from build123d import *

# Parameters (mm, degrees)
F0_R     = 8
F1_DEPTH = 3.5
F2_R     = 12.5
F2_R_2   = 8
F3_DEPTH = 1
F4_W     = 20
F4_H     = 2
F5_DEPTH = 2
F6_W     = 1.5
F6_H     = 3
F7_DEPTH = 0.25


with BuildPart() as f1:
    # F0 (on Top) → F1 (new body)
    with BuildSketch(Plane.XY):
        with BuildLine():
            ThreePointArc((0, -12.5), (8.838835, -8.838835), (12.5, 0))
            ThreePointArc((12.5, 0), (8.838835, 8.838835), (0, 12.5))
            ThreePointArc((0, 12.5), (-12.5, 0), (0, -12.5))
        make_face()
        Circle(F0_R, mode=Mode.SUBTRACT)
        with BuildLine():
            ThreePointArc((0, -12.5), (-12.5, 0), (0, 12.5))
            Line((0, 12.5), (-35, 12.5))
            Line((-35, 12.5), (-116.388784, 2.506714))
            Line((-116.388784, 2.506714), (-116.388784, -2.506714))
            Line((-116.388784, -2.506714), (-35, -12.5))
            Line((-35, -12.5), (0, -12.5))
        make_face()
    extrude(amount=F1_DEPTH)

    # F2 (on face) → F3 (join)
    with BuildSketch(Plane.XY.offset(3.5)):
        Circle(F2_R)
        Circle(F2_R_2, mode=Mode.SUBTRACT)
    extrude(amount=F3_DEPTH)

    # F4 (on face) → F5 (cut)
    with BuildSketch(Plane.XY.offset(3.5)):
        with Locations((-106.388784, -0.006714)):
            Rectangle(F4_W, F4_H)
    extrude(amount=-F5_DEPTH, mode=Mode.SUBTRACT)

    # F6 (on face) → F7 (join)
    with BuildSketch(Plane.XY.offset(4.5)):
        with Locations((0, 10.153166)):
            Rectangle(F6_W, F6_H)
        Polygon((3.237552, 11.219494), (1.772621, 11.541949), (1.127709, 8.612088), (2.59264, 8.289632), align=None)
        Polygon((5.573719, 10.26121), (4.212356, 10.891044), (2.952689, 8.168318), (4.314052, 7.538484), align=None)
        Polygon((7.649265, 8.823124), (6.455126, 9.730885), (4.639603, 7.342606), (5.833743, 6.434845), align=None)
        Polygon((9.367141, 6.972478), (8.396061, 8.115721), (6.109575, 6.173563), (7.080655, 5.030319), align=None)
        Polygon((10.647019, 4.795807), (9.944406, 6.121075), (7.29387, 4.71585), (7.996483, 3.390582), align=None)
        Polygon((11.429054, 2.39489), (11.027762, 3.840215), (8.137112, 3.03763), (8.538404, 1.592305), align=None)
        Polygon((11.67668, -0.11801), (11.595471, 1.37979), (8.599871, 1.217373), (8.68108, -0.280427), align=None)
        Polygon((11.378317, -2.625392), (11.62099, -1.145153), (8.66051, -0.659807), (8.417837, -2.140046), align=None)
        Polygon((10.547916, -5.010014), (11.103124, -3.616549), (8.316193, -2.506134), (7.760986, -3.899599), align=None)
        Polygon((9.224307, -7.160373), (10.066088, -5.918839), (7.583021, -4.235278), (6.74124, -5.476812), align=None)
        Polygon((7.469379, -8.975921), (8.558373, -7.944371), (6.495274, -5.766385), (5.406281, -6.797934), align=None)
        Polygon((5.365192, -10.371764), (6.650478, -9.598434), (5.103816, -7.027862), (3.81853, -7.801193), align=None)
        Polygon((3.010134, -11.282636), (4.431614, -10.803684), (3.473709, -7.960724), (2.052229, -8.439676), align=None)
        Polygon((0.514325, -11.665944), (2.005532, -11.503765), (1.681175, -8.521352), (0.189968, -8.68353), align=None)
        Polygon((-2.005532, -11.503765), (-0.514325, -11.665944), (-0.189968, -8.68353), (-1.681175, -8.521352), align=None)
        Polygon((-4.431614, -10.803684), (-3.010134, -11.282636), (-2.052229, -8.439676), (-3.473709, -7.960724), align=None)
        Polygon((-6.650478, -9.598434), (-5.365192, -10.371764), (-3.81853, -7.801193), (-5.103816, -7.027862), align=None)
        Polygon((-8.558373, -7.944371), (-7.469379, -8.975921), (-5.406281, -6.797934), (-6.495274, -5.766385), align=None)
        Polygon((-10.066088, -5.918839), (-9.224307, -7.160373), (-6.74124, -5.476812), (-7.583021, -4.235278), align=None)
        Polygon((-11.103124, -3.616549), (-10.547916, -5.010014), (-7.760986, -3.899599), (-8.316193, -2.506134), align=None)
        Polygon((-11.62099, -1.145153), (-11.378317, -2.625392), (-8.417837, -2.140046), (-8.66051, -0.659807), align=None)
        Polygon((-11.595471, 1.37979), (-11.67668, -0.11801), (-8.68108, -0.280427), (-8.599871, 1.217373), align=None)
        Polygon((-11.027762, 3.840215), (-11.429054, 2.39489), (-8.538404, 1.592305), (-8.137112, 3.03763), align=None)
        Polygon((-9.944406, 6.121075), (-10.647019, 4.795807), (-7.996483, 3.390582), (-7.29387, 4.71585), align=None)
        Polygon((-8.396061, 8.115721), (-9.367141, 6.972478), (-7.080655, 5.030319), (-6.109575, 6.173563), align=None)
        Polygon((-6.455126, 9.730885), (-7.649265, 8.823124), (-5.833743, 6.434845), (-4.639603, 7.342606), align=None)
        Polygon((-4.212356, 10.891044), (-5.573719, 10.26121), (-4.314052, 7.538484), (-2.952689, 8.168318), align=None)
        Polygon((-1.772621, 11.541949), (-3.237552, 11.219494), (-2.59264, 8.289632), (-1.127709, 8.612088), align=None)
    extrude(amount=F7_DEPTH)


solid = f1.part
Could you check a few things on this model? Use its own coordinates, in mm. A direction names the side the tool comes from. Coordinates: 2 decimals unless noted, no trailing zeros. Loops run counter-clockwise (first coordinate to the right, second up) from the corner with the lowest first, then second, coordinate; pieces in that order, holes last.
1. Imagine slicing it at A-A (x = -52). Please give me the cut outline in (y, z).
2. I need wall thicknesses on L1, parallel to Y at x = -99, z = 1.8; L2, parallel to Y at x = 0, z = 1.95; L3, parallel to Z at x = -60, y = 5.75. Which ranges of each line are inside material? Lowest first, please.
3. For faces 1 (the face through (-107, -1.007, 3)), 2 (the face through (3, -10, 4.75)), which set-ups out of +Z, -Z, +X, -X, +Y, -Y let a thin tool reach every point of the face, with its end or its side?
4. For P1, Ø1.6, axis at x = -104.5, z = 2.5, coming from the -Y side; P2, Ø5, axis at x = -98, y = -3, coming from the +Z side; P3, Ø1.6, axis at x = -108.5, y = 0, coming from the +Z side, each with a flat end and sliding along its axis, tell me the tip position at first contact or that it passes through.
5. We'd pull the mould along X, two halves only. Please class faces 3 (the face through (-1.73, -7.81, 2.22)), 4 (the face through (-10, 3, 4.75)), 5 (the face through (-76.264, -7.433, 1.726)): released by +X, released by -X, zero draft, split by the parting line, or undercut.
Computed values:
1. outline: (-10.41, 0) - (10.41, 0) - (10.41, 3.5) - (-10.41, 3.5) - close
2. L1: y = -4.64 to -1.01, 0.99 to 4.64
2. L2: y = -12.5 to -8, 8 to 12.5
2. L3: z = 0 to 3.5
3. face 1: +Z, -X
3. face 2: +Z, +X, -X, +Y, -Y
4. P1: stops at y = -4.06
4. P2: stops at z = 3.5
4. P3: stops at z = 1.5
5. face 3: undercut
5. face 4: zero draft
5. face 5: released by -X
